Build history of the part. All positions in model axes, mm. Give positions to 0.01 mm unless a question says otherwise; leave off trailing zeros. Order: outer loops, then holes, each group sorted by start corner. A loop starts at its lowest first (then second) coordinate and runs counter-clockwise, first axis right, second up. Notation, with made-up numbers: (-22.5, -30.5) -> (9.5, -30.5) arc R29 cw to (9.5, 5.5) -> close; hole circle Ø1 at (76, 8). An arc over 180 degrees is marked (long way). One line per item, written item: value. Start each with the question number.
(1) Saw through at B-B on z = 0.45. Count the separate pieces of the cut face and the enclosed holes in it, plus the area to 3 significant figures.
(2) Saw through at C-C on x = 40. Give the cut face in (y, z), plus the area to 3 significant figures.
(3) Saw through at A-A on y = 2.5. Give the cut face in (x, z).
(4) Probe line 1 (Y direction, x = 2.5, z = 0.85); line 2 (Y direction, x = 31, z = 0.85); line 3 (X direction, y = 8.75, z = 0.55). List the from-to ranges inside material, lowest first.
(5) Saw through at D-D on y = 24.5. Give the cut face in (x, z).
```python
from build123d import *

# Parameters (mm, degrees)
ESQUISSE1_R        = 1.75
BOSS_EXTRU_1_DEPTH = 1.5
CONG_1_R           = 2


with BuildPart() as part:
    # Esquisse1 → Boss.-Extru.1 (new body)
    with BuildSketch(Plane.XY):
        with BuildLine():
            Line((0, 0), (27, 0))
            Line((27, 0), (27, 18))
            Line((27, 18), (42, 18))
            ThreePointArc((42, 18), (44.5, 20.5), (42, 23))
            Line((42, 23), (27, 23))
            Line((27, 23), (27, 27))
            Line((27, 27), (0, 27))
            Line((0, 27), (0, 0))
        make_face()
        with Locations((2.5, 24.5)):
            Circle(ESQUISSE1_R, mode=Mode.SUBTRACT)
        with Locations((24.5, 2.5)):
            Circle(ESQUISSE1_R, mode=Mode.SUBTRACT)
    extrude(amount=BOSS_EXTRU_1_DEPTH)

    # Congé1
    cong_1_edges = [part.edges().sort_by_distance(p)[0] for p in [
        (27, 23, 0.75),
        (27, 18, 0.75),
        (27, 0, 0.75),
        (0, 0, 0.75),
        (0, 27, 0.75),
        (27, 27, 0.75),
    ]]
    fillet(cong_1_edges, radius=CONG_1_R - 0.0001)  # a hair under: the kernel refuses the full size


solid = part.part
```
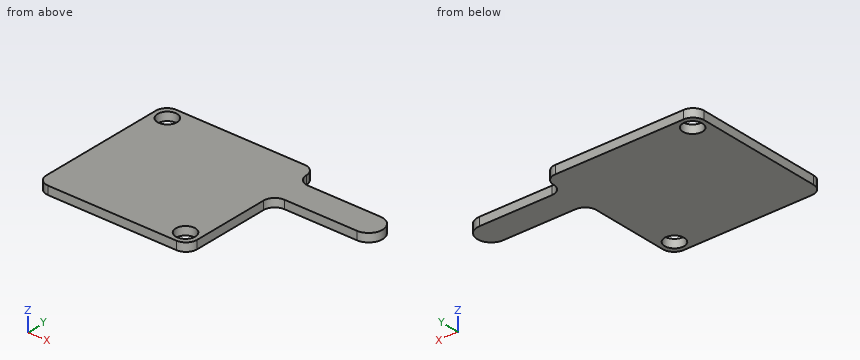
Results below:
1. separate pieces: 1
1. enclosed holes: 2
1. area: 793 mm²
2. outline: (18, 0) -> (23, 0) -> (23, 1.5) -> (18, 1.5) -> close
2. area: 7.50 mm²
3. outline: (0, 0) -> (22.75, 0) -> (22.75, 1.5) -> (0, 1.5) -> close; (26.25, 0) -> (27, 0) -> (27, 1.5) -> (26.25, 1.5) -> close
4. line 1: y = 0 to 22.75, 26.25 to 27
4. line 2: y = 18 to 23
4. line 3: x = 0 to 27
5. outline: (0, 0) -> (0.75, 0) -> (0.75, 1.5) -> (0, 1.5) -> close; (4.25, 0) -> (27.06, 0) -> (27.06, 1.5) -> (4.25, 1.5) -> close
